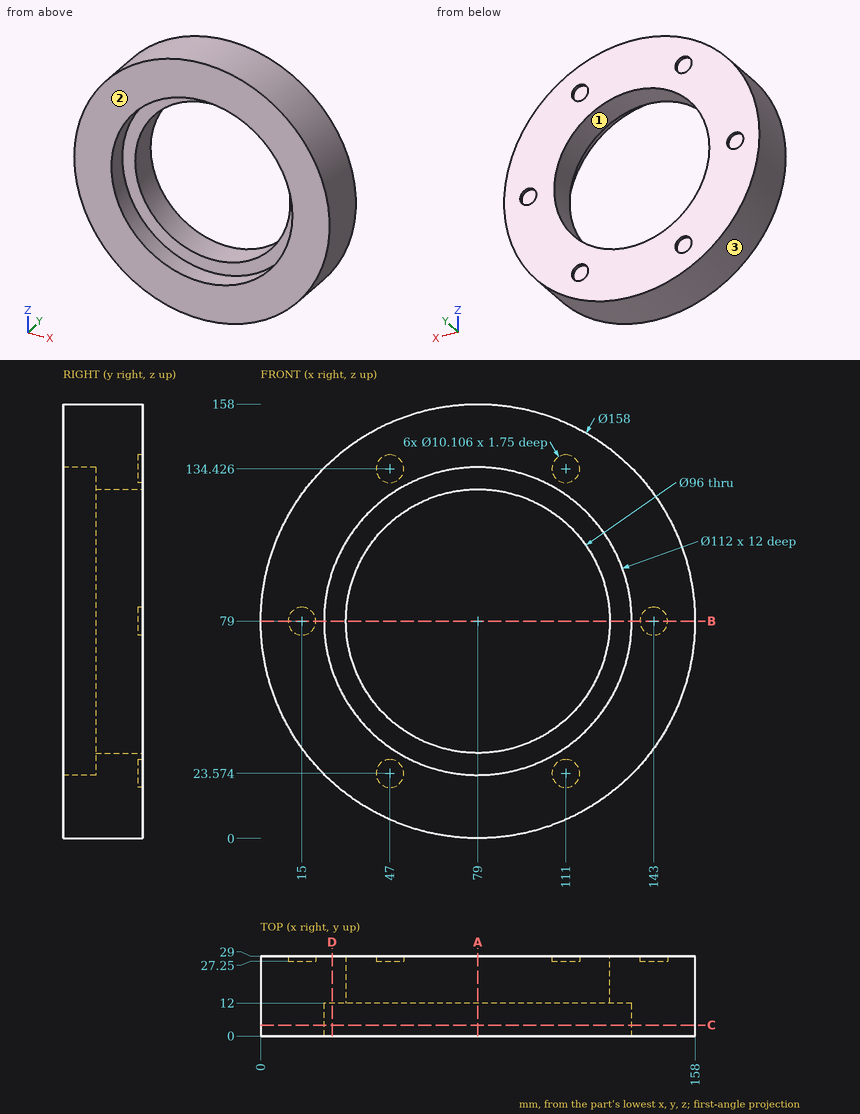
The drawing under review shows one solid part. Ordinate dimensions are in mm from its lowest x, y, z. Coordinates: 2 decimals unless noted, no trailing zeros. Loops run counter-clockwise (first coordinate to the right, second up) from the corner with the lowest first, then second, coordinate; pieces in that order, holes last. Notation, with made-up numbers: (-10.75, 57.5) -> (17.25, 57.5) arc R25 cw to (17.25, 92.5) -> close; hole circle Ø3 at (87.25, -21.75). An arc over 180 degrees is marked (long way). Answer as a JSON object with one key per item and string values.
Q1. The part is to be moulded in two halves that separate along Z. For the marked faces 1, 2 and 3, say which applies: +Z half, -Z half, draft (parallel to the pull), parting line (faces both ways), or undercut.
Answer block:
{"face 1": "undercut", "face 2": "draft", "face 3": "parting line"}
Q2. Take a section at B-B on z = 79. Give the boundary of the cut face in (x, y).
Answer block:
{"outline": "(0, 0) -> (23, 0) -> (23, 12) -> (31, 12) -> (31, 29) -> (20.05, 29) -> (20.05, 27.25) -> (9.95, 27.25) -> (9.95, 29) -> (0, 29) -> close; (127, 12) -> (135, 12) -> (135, 0) -> (158, 0) -> (158, 29) -> (148.05, 29) -> (148.05, 27.25) -> (137.95, 27.25) -> (137.95, 29) -> (127, 29) -> close"}
Q3. Take a section at D-D on x = 26. Give the boundary of the cut face in (y, z).
Answer block:
{"outline": "(0, 20.42) -> (29, 20.42) -> (29, 137.58) -> (0, 137.58) -> (0, 97.08) -> (12, 97.08) -> (12, 60.92) -> (0, 60.92) -> close"}
Q4. Take a section at C-C on y = 4. Give the boundary of the cut face in (x, z).
Answer block:
{"outline": "circle Ø158 at (79, 79); hole circle Ø112 at (79, 79)"}
Q5. Take a section at A-A on x = 79. Give the boundary of the cut face in (y, z).
Answer block:
{"outline": "(0, 0) -> (29, 0) -> (29, 31) -> (12, 31) -> (12, 23) -> (0, 23) -> close; (0, 135) -> (12, 135) -> (12, 127) -> (29, 127) -> (29, 158) -> (0, 158) -> close"}
Q6. To check wall thickness, follow L1, parallel to Z at x = 111, y = 28.15 (1 decimal); L2, parallel to Z at x = 79, y = 15.5; L3, parallel to Y at x = 121.5, z = 48. State the ranges of each line that lie inside material, in increasing order.
Answer block:
{"L1": "z = 6.8 to 18.5, 28.6 to 43.2, 114.8 to 129.4, 139.5 to 151.2", "L2": "z = 0 to 31, 127 to 158", "L3": "y = 12 to 29"}
Q7. Clearance check with flat-ended pins moving along their axes: pin 1 Ø3 at (x, z) = (113, 133) entering from +Y; pin 2 Ø1.5 at (x, y) = (135, 19.5) entering from +Z (1 decimal); pin 3 Ø4 at (y, z) = (24.5, 49) entering from +X. State where each tip first meets the part, or that it passes through.
Answer block:
{"pin 1": "stops at y = 27.25", "pin 2": "stops at z = 135.5", "pin 3": "stops at x = 152.87"}
